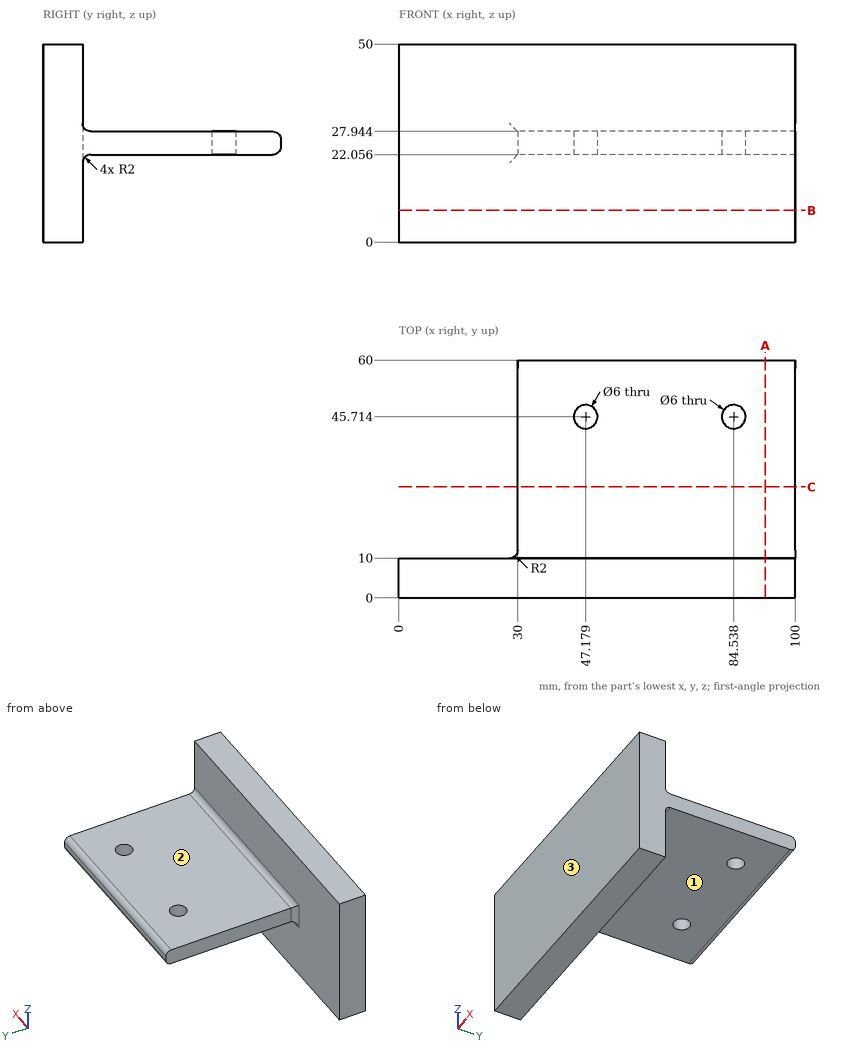
Geometry: see drawing. Coordinates: mm, zero at the bounding-box minimum. A direction names the side the tool comes from. Coordinates: 2 decimals unless noted, no trailing zeros. Loops run counter-clockwise (first coordinate to the right, second up) from the corner with the lowest first, then second, coordinate; pieces in that order, holes last.
Q1. Cut plane A-A (x = 92.5). Output: boundary loops of the cut face in (y, z).
Q2. Contact query for flat-ended pins moving along their axis: pin 1 (8 mm diameter, centred on x = 29, y = 45, fed in from +Z); pin 2 (8 mm diameter, centred on y = 31.5, z = 19, fed in from -X); pin 3 (7 mm diameter, centred on x = 84.54, y = 45.71, fed in from -Z); pin 4 (1.5 mm diameter, centred on x = 65.5, z = 38.5, fed in from -Y). Output: stop coordinate, or through.
Q3. Cut plane B-B (z = 8). Output: boundary loops of the cut face in (x, y).
Q4. Cut plane C-C (y = 28). Output: boundary loops of the cut face in (x, z), then the cut area to 3 significant figures.
Q5. Set-up query: the marked faces 1, 2 and 3. Return all of +Z, -Z, +X, -X, +Y, -Y with unobstructed straight access to the full face (end or side cutting, diameter ignored); none if empty.
Q6. Material intervals for line 1 (Y direction, x = 39, z = 10.5); line 2 (Z direction, x = 66, y = 39.5); line 3 (Y direction, x = 48, z = 25.5), sorted ascending.
Working result:
1. outline: (0, 0) - (10, 0) - (10, 20.06) arc R2 cw to (12, 22.06) - (58, 22.06) arc R2 ccw to (60, 24.06) - (60, 25.94) arc R2 ccw to (58, 27.94) - (12, 27.94) arc R2 cw to (10, 29.94) - (10, 50) - (0, 50) - close
2. pin 1: stops at z = 27.94
2. pin 2: stops at x = 30
2. pin 3: stops at z = 22.06
2. pin 4: stops at y = 0
3. outline: (0, 0) - (100, 0) - (100, 10) - (0, 10) - close
4. outline: (30, 22.06) - (100, 22.06) - (100, 27.94) - (30, 27.94) - close
4. area: 412 mm2
5. face 1: -Z, +X, -X, +Y
5. face 2: +Z, +X, -X, +Y
5. face 3: +Z, -Z, +X, -X, -Y
6. line 1: y = 0 to 10
6. line 2: z = 22.06 to 27.94
6. line 3: y = 0 to 42.83, 48.6 to 60
